The listing builds one solid part. Answer for the finished solid, in the listing's coordinates (mm). Give positions to 0.01 mm unless a question says otherwise; leave off trailing zeros. Order: outer loops, then holes, each group sorted by start corner. A loop starts at its lowest first (then second) coordinate and runs counter-clockwise, first axis right, second up. Notation, with made-up numbers: (74.5, 75.25) - (120.5, 75.25) arc R20 cw to (120.5, 94.25) - close; hole circle Ø8 at (-11.75, -31). An arc over 180 degrees is marked (long way). Use a Markdown table: item, result. Add a question column.
1) Straight lines are drawn through the part: line 1 (Y direction, x = 11.5, z = 5); line 2 (Z direction, x = 9.25, y = 3.25); line 3 (Z direction, x = 4, y = 2.5). For each, find the intervals that lie inside material, in ascending order.
2) Find section B-B, the plane y = 2.5. Determine the outline of the cut face in (x, z), plus the area to 3 significant figures.
3) Find section A-A, the plane z = 5.25. Determine the outline of the cut face in (x, y), plus the area to 4 significant figures.
4) The mould has two halves that part along Y. Classify faces 1 (the face through (6.409, 3.798, 4.852)), 2 (the face through (6.409, 7.554, 5.027)), 3 (the face through (6, 3, 9.899)): released by +Y, released by -Y, zero draft, split by the parting line, or undercut.
5) Find section D-D, the plane y = 5.75. Determine the outline of the cut face in (x, z), plus the area to 3 significant figures.
6) Find section C-C, the plane x = 10.75. Determine the outline of the cut face in (y, z).
7) Flat-ended cylindrical pins translate along their axes: pin 1 (1 mm diameter, centred on y = 4.5, z = 8, fed in from -X); pin 2 (1 mm diameter, centred on x = 2.5, z = 6.5, fed in from +Y). Find the tip coordinate at first contact, or state that the pin passes through.
from build123d import *

# Parameters (mm, degrees)
BOSS_EXTRUDE1_DEPTH   = 13
F_1_5MM_DOWEL_SLOT1_D = 1.5


with BuildPart() as part:
    # Sketch1 → Boss-Extrude1 (new body)
    with BuildSketch(Plane(origin=(0, 0, 0), x_dir=(0, 0, -1), z_dir=(1, 0, 0))):
        with BuildLine():
            Line((0, 0), (-9.899494937, 0))
            Line((-9.899494937, 0), (-9.899494937, 5.503823677))
            ThreePointArc((-9.899494937, 5.503823677), (-4.949747468, 7.554076209), (0, 5.503823677))
            Line((0, 5.503823677), (0, 0))
        make_face()
    extrude(amount=BOSS_EXTRUDE1_DEPTH)

    # Ø1.5mm Dowel Slot1 (through all)
    with Locations(Plane(origin=(13, 0, 0), x_dir=(0, 0, -1), z_dir=(1, 0, 0))):
        with Locations((-4.949747468, 3.054076209)):
            Hole(F_1_5MM_DOWEL_SLOT1_D / 2)


solid = part.part
The answers:
| question | item | result |
|---|---|---|
| 1 | line 1 | 0 to 2.31, 3.8 to 7.55 |
| 1 | line 2 | 0 to 4.23, 5.67 to 9.9 |
| 1 | line 3 | 0 to 4.44, 5.46 to 9.9 |
| 2 | outline | (0, 0) - (13, 0) - (13, 4.44) - (0, 4.44) - close; (0, 5.46) - (13, 5.46) - (13, 9.9) - (0, 9.9) - close |
| 2 | area | 116 mm2 |
| 3 | outline | (0, 0) - (13, 0) - (13, 2.37) - (0, 2.37) - close; (0, 3.74) - (13, 3.74) - (13, 7.55) - (0, 7.55) - close |
| 3 | area | 80.25 mm2 |
| 4 | face 1 | undercut |
| 4 | face 2 | released by +Y |
| 4 | face 3 | zero draft |
| 5 | outline | (0, 0.26) - (13, 0.26) - (13, 9.64) - (0, 9.64) - close |
| 5 | area | 122 mm2 |
| 6 | outline | (0, 0) - (5.5, 0) arc R7 ccw to (5.5, 9.9) - (0, 9.9) - close; hole circle Ø1.5 at (3.05, 4.95) |
| 7 | pin 1 | x = 0 |
| 7 | pin 2 | y = 7.47 |
